Verification items for the finished model (mm, model axes). Face numbers are marked on the shaded views. A direction names the side the tool comes from. Round coordinates to 2 decimals unless told otherwise and drop trailing zeros. Order: outer loops, then holes, each group sorted by start corner. A loop starts at its lowest first (then second) coordinate and runs counter-clockwise, first axis right, second up.
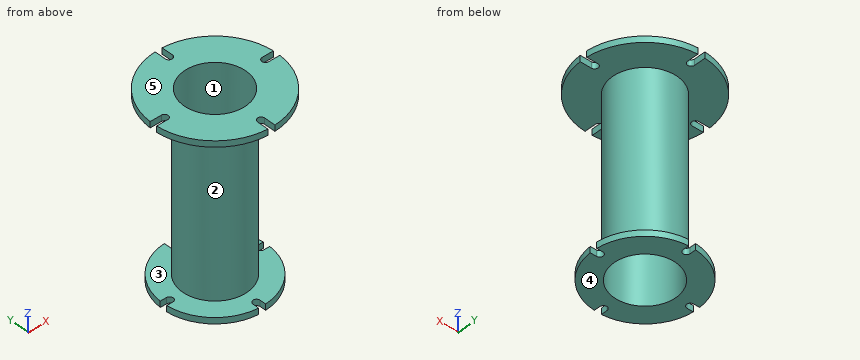
```python
from build123d import *

# Parameters (mm, degrees)
F0_R     = 64
F0_R_2   = 61
F1_DEPTH = 360
F2_R     = 64
F3_DEPTH = 12
F4_R     = 64
F5_DEPTH = 12


with BuildPart() as f1:
    # F0 (on Top) → F1 (new body)
    with BuildSketch(Plane.XY):
        Circle(F0_R)
        Circle(F0_R_2, mode=Mode.SUBTRACT)
    extrude(amount=F1_DEPTH)

    # F2 (on face) → F3 (join)
    with BuildSketch(Plane.XY.offset(360)):
        with BuildLine():
            Line((-100, -7), (-122.299836, -7))
            ThreePointArc((-122.299836, -7), (-86.620581, -86.620581), (-7, -122.299836))
            Line((-7, -122.299836), (-7, -100))
            ThreePointArc((-7, -100), (0, -93), (7, -100))
            Line((7, -100), (7, -122.299836))
            ThreePointArc((7, -122.299836), (86.620581, -86.620581), (122.299836, -7))
            Line((122.299836, -7), (100, -7))
            ThreePointArc((100, -7), (93, 0), (100, 7))
            Line((100, 7), (122.299836, 7))
            ThreePointArc((122.299836, 7), (86.620581, 86.620581), (7, 122.299836))
            Line((7, 122.299836), (7, 100))
            ThreePointArc((7, 100), (0, 93), (-7, 100))
            Line((-7, 100), (-7, 122.299836))
            ThreePointArc((-7, 122.299836), (-86.620581, 86.620581), (-122.299836, 7))
            Line((-122.299836, 7), (-100, 7))
            ThreePointArc((-100, 7), (-93, 0), (-100, -7))
        make_face()
        Circle(F2_R, mode=Mode.SUBTRACT)
    extrude(amount=-F3_DEPTH)

    # F4 (on face) → F5 (join)
    with BuildSketch(Plane(origin=(0, 0, 0), x_dir=(1, 0, 0), z_dir=(0, 0, -1))):
        with BuildLine():
            Line((-7, 90), (-7, 102.260696))
            ThreePointArc((-7, 102.260696), (-72.478445, 72.478445), (-102.260696, 7))
            Line((-102.260696, 7), (-90, 7))
            ThreePointArc((-90, 7), (-83, 0), (-90, -7))
            Line((-90, -7), (-102.260696, -7))
            ThreePointArc((-102.260696, -7), (-72.478445, -72.478445), (-7, -102.260696))
            Line((-7, -102.260696), (-7, -90))
            ThreePointArc((-7, -90), (0, -83), (7, -90))
            Line((7, -90), (7, -102.260696))
            ThreePointArc((7, -102.260696), (72.478445, -72.478445), (102.260696, -7))
            Line((102.260696, -7), (90, -7))
            ThreePointArc((90, -7), (83, 0), (90, 7))
            Line((90, 7), (102.260696, 7))
            ThreePointArc((102.260696, 7), (72.478445, 72.478445), (7, 102.260696))
            Line((7, 102.260696), (7, 90))
            ThreePointArc((7, 90), (0, 83), (-7, 90))
        make_face()
        Circle(F4_R, mode=Mode.SUBTRACT)
    extrude(amount=-F5_DEPTH)


solid = f1.part
```
1) Sectioned sample at C-C on z = 78.5. Record the cut outline in (x, y).
2) Sectioned sample at A-A on y = 0. Record the cut outline in (x, z).
3) Tool access check on the marked faces 1 and 2. Record the directions out of +Z, -Z, +X, -X, +Y, -Y that give a thin tool (end or side, any length) a straight path to the whole face; none if there is none.
4) Draft check along Z on the marked faces 3, 4 and 5. Enter one of: released by +Z, released by -Z, zero draft, split by the parting line, or undercut.
5) Scan lines: probe 1 along Y at (x, z) = (0, 279); probe 2 along Z at (x, y) = (89.5, -16); probe 3 along Y at (x, z) = (53, 254.5). Record each from-to range of solid material in increasing order.
6) Sectioned sample at B-B on x = 71.5. Record the cut outline in (y, z), then the cut area to 3 significant figures.
7) Go/stop test with flat-tipped pins: pin 1 Ø3 at (y, z) = (17, 188.5) entering from -X; pin 2 Ø6 at (x, z) = (95, 8.5) entering from -Y; pin 3 Ø3.5 at (y, z) = (-96, 5.5) entering from +X; pin 4 Ø4 at (x, y) = (-65.5, 33) entering from -Z. Record where each tip stops, or that it passes through.
8) Sectioned sample at D-D on y = -37. Record the cut outline in (x, z).
Returned:
1. outline: circle Ø128 at (0, 0); hole circle Ø122 at (0, 0)
2. outline: (-93, 348) - (-64, 348) - (-64, 12) - (-83, 12) - (-83, 0) - (-61, 0) - (-61, 360) - (-93, 360) - close; (61, 0) - (83, 0) - (83, 12) - (64, 12) - (64, 348) - (93, 348) - (93, 360) - (61, 360) - close
3. face 1: +Z, -Z
3. face 2: none
4. face 3: undercut
4. face 4: released by -Z
4. face 5: released by +Z
5. probe 1: y = -64 to -61, 61 to 64
5. probe 2: z = 0 to 12, 348 to 360
5. probe 3: y = -35.87 to -30.2, 30.2 to 35.87
6. outline: (-99.47, 348) - (99.47, 348) - (99.47, 360) - (-99.47, 360) - close; (-73.44, 0) - (73.44, 0) - (73.44, 12) - (-73.44, 12) - close
6. area: 4,150 mm2
7. pin 1: stops at x = -62.09
7. pin 2: stops at y = -45.19
7. pin 3: stops at x = 40.29
7. pin 4: stops at z = 0
8. outline: (-116.78, 348) - (-52.22, 348) - (-52.22, 12) - (-95.59, 12) - (-95.59, 0) - (-48.5, 0) - (-48.5, 360) - (-116.78, 360) - close; (48.5, 0) - (95.59, 0) - (95.59, 12) - (52.22, 12) - (52.22, 348) - (116.78, 348) - (116.78, 360) - (48.5, 360) - close
